Check sheet for the modelled part. Datum: model origin and axes. Units: mm. A direction names the side the tool comes from. Round coordinates to 2 decimals unless told otherwise and drop trailing zeros. Loops run counter-clockwise (first coordinate to the right, second up) from the corner with the lowest first, then second, coordinate; pieces in that order, holes last. Notation, with made-up numbers: (39.25, 68.25) -> (94.25, 68.25) arc R26 ccw to (94.25, 100.25) -> close; hole circle Ø9 at (3.5, -39). An arc over 180 degrees is marked (long way). Return JSON: item names as keys, results as strings.
from build123d import *

# Parameters (mm, degrees)
F0_W     = 30
F0_H     = 35
F1_DEPTH = 3
F2_W     = 18
F2_H     = 15
F3_DEPTH = 35
F4_R     = 6
F5_DEPTH = 40
F6_R     = 1.5
F7_DEPTH = 25


with BuildPart() as f1:
    # F0 (on Top) → F1 (new body)
    with BuildSketch(Plane.XY):
        Rectangle(F0_W, F0_H)
    extrude(amount=F1_DEPTH)

    # F2 (on face) → F3 (join)
    with BuildSketch(Plane.XZ.offset(17.5)):
        with Locations((0, 10.5)):
            Rectangle(F2_W, F2_H)
    extrude(amount=-F3_DEPTH)

    # F4 (on face) → F5 (cut)
    with BuildSketch(Plane.XZ.offset(17.5)):
        with Locations((0, 10.5)):
            Circle(F4_R)
    extrude(amount=-F5_DEPTH, mode=Mode.SUBTRACT)

    # F6 (on face) → F7 (cut)
    with BuildSketch(Plane.XY.offset(3)):
        with Locations((12, 12.5)):
            Circle(F6_R)
        with Locations((12, -12.5)):
            Circle(F6_R)
        with Locations((-12, -12.5)):
            Circle(F6_R)
        with Locations((-12, 12.5)):
            Circle(F6_R)
    extrude(amount=-F7_DEPTH, mode=Mode.SUBTRACT)


solid = f1.part
Q1. Section check A-A (y = -12.5). Record the boundary of the cut face in (x, z), then the cut area to 3 significant figures.
Results list:
{"outline": "(-15, 0) -> (-13.5, 0) -> (-13.5, 3) -> (-15, 3) -> close; (-10.5, 0) -> (10.5, 0) -> (10.5, 3) -> (9, 3) -> (9, 18) -> (-9, 18) -> (-9, 3) -> (-10.5, 3) -> close; (13.5, 0) -> (15, 0) -> (15, 3) -> (13.5, 3) -> close; hole circle Ø12 at (0, 10.5)", "area": "229 mm^2"}
Q2. Tool access check on faces 1 (the flat face through (9, 0, 10)), 2 (the flat face through (-12, 0, 3)), 3 (the flat face through (0, 0, 18)). Record the directions out of +Z, -Z, +X, -X, +Y, -Y that give a thin tool (end or side, any length) a straight path to the whole face; none if there is none.
Results list:
{"face 1": "+Z, +X, +Y, -Y", "face 2": "+Z, -X, +Y, -Y", "face 3": "+Z, +X, -X, +Y, -Y"}
Q3. Section check C-C (x = 0). Record the boundary of the cut face in (y, z), then the cut area to 3 significant figures.
Results list:
{"outline": "(-17.5, 0) -> (17.5, 0) -> (17.5, 4.5) -> (-17.5, 4.5) -> close; (-17.5, 16.5) -> (17.5, 16.5) -> (17.5, 18) -> (-17.5, 18) -> close", "area": "210 mm^2"}
Q4. Go/stop test with flat-tipped pins: pin 1 (6.5 mm diameter, centred on x = 13, y = -3, fed in from +Z); pin 2 (7.5 mm diameter, centred on y = 8, z = 10, fed in from -X). Record where each tip stops, or that it passes through.
Results list:
{"pin 1": "z = 3", "pin 2": "x = -9"}
Q5. Section check B-B (x = -12). Record the boundary of the cut face in (y, z), then the cut area to 3 significant figures.
Results list:
{"outline": "(-17.5, 0) -> (-14, 0) -> (-14, 3) -> (-17.5, 3) -> close; (-11, 0) -> (11, 0) -> (11, 3) -> (-11, 3) -> close; (14, 0) -> (17.5, 0) -> (17.5, 3) -> (14, 3) -> close", "area": "87.0 mm^2"}
Q6. Material ranges on line 1 (Y direction, x = -12, z = 2.1); line 2 (Z direction, x = -10.5, y = -13.5); line 3 (X direction, y = -13, z = 1.5), recorded low to high.
Results list:
{"line 1": "-17.5 to -14, -11 to 11, 14 to 17.5", "line 2": "0 to 3", "line 3": "-15 to -13.41, -10.59 to 10.59, 13.41 to 15"}
Q7. Draft check along Y on faces 4 (the flat face through (-4, 17.5, 5)), 5 (the flat face through (-9, 0, 10)), 6 (the cylindrical face through (10.5, 12.57, 1.52)). Enter one of: released by +Y, released by -Y, zero draft, split by the parting line, or undercut.
Results list:
{"face 4": "released by +Y", "face 5": "zero draft", "face 6": "undercut"}
Q8. Section check D-D (z = 10.5). Record the boundary of the cut face in (x, y).
Results list:
{"outline": "(-9, -17.5) -> (-6, -17.5) -> (-6, 17.5) -> (-9, 17.5) -> close; (6, -17.5) -> (9, -17.5) -> (9, 17.5) -> (6, 17.5) -> close"}
